from build123d import *

# Parameters (mm, degrees)
CUT_EXTRUDE1_DEPTH = 1.1


with BuildPart() as part:
    # Sketch1 → Revolve1 (revolve)
    with BuildSketch(Plane.XY):
        with BuildLine():
            Line((-2.36, 0), (-2.36, 2))
            Line((-2.36, 2), (-2.11, 2.25))
            Line((-2.11, 2.25), (0, 2.25))
            Line((0, 2.25), (0, 1.35))
            ThreePointArc((0, 1.35), (0.029289322, 1.279289322), (0.1, 1.25))
            Line((0.1, 1.25), (9.7565, 1.25))
            Line((9.7565, 1.25), (10, 1.0065))
            Line((10, 1.0065), (10, 0))
            Line((10, 0), (-2.36, 0))
        make_face()
    revolve(axis=Axis((10, 0, 0), (-1, 0, 0)))

    # Sketch2 → Cut-Extrude1 (cut)
    with BuildSketch(Plane(origin=(-2.36, 0, 0), x_dir=(0, 0, -1), z_dir=(1, 0, 0))):
        Polygon((-1, 0.577350269), (-1, -0.577350269), (0, -1.154700538), (1, -0.577350269), (1, 0.577350269), (0, 1.154700538), align=None)
    extrude(amount=CUT_EXTRUDE1_DEPTH, mode=Mode.SUBTRACT)

    # Sketch3 → Cut-Revolve1 (revolve, cut)
    with BuildSketch(Plane.XY):
        Polygon((-1.26, 0), (-1.26, 1), (-0.682649731, 0), align=None)
    revolve(axis=Axis((-0.682649731, 0, 0), (-1, 0, 0)), mode=Mode.SUBTRACT)


solid = part.part
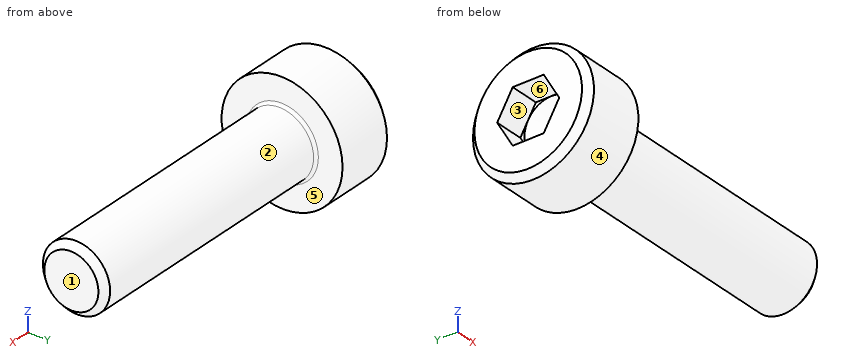
Could you check a few things on this model? Use its own coordinates, in mm. Face numbers are marked on the shaded views. A direction names the side the tool comes from. Round coordinates to 2 decimals unless told otherwise and drop trailing zeros. Write each loop counter-clockwise with the first axis right and the second up, starting at its lowest first coordinate (ties: lowest second). Pieces come first, ordered by that corner, then holes. Notation, with made-up numbers: (69.25, -28) -> (114.25, -28) arc R16 ccw to (114.25, -9) -> close; hole circle Ø7 at (31, 46.5). An arc over 180 degrees is marked (long way). Use a Markdown table: item, result.
1. Please list where these lines run through material, in increasing order: probe 1 along X at (y, z) = (0.8, 1.4); probe 2 along Z at (x, y) = (3.25, 0); probe 3 along Y at (x, z) = (-1.5, 0.15) (3 decimals).
Answer key:
| item | result |
|---|---|
| probe 1 | x = -2.36 to 0 |
| probe 2 | z = -1.25 to 1.25 |
| probe 3 | y = -2.245 to -1.068, 1.068 to 2.245 |
2. If we section it at A-A (x = 1): List the corners of the cut face in (y, z) for me.
Answer key:
| item | result |
|---|---|
| outline | circle Ø2.5 at (0, 0) |
3. Which directions (+Z, -Z, +X, -X, +Y, -Y) give clear straight access to the entire face, cutting with the end or side of a thin tool? Please do the marked faces 4, 5 and 6.
Answer key:
| item | result |
|---|---|
| face 4 | +X, -X |
| face 5 | +X |
| face 6 | -X |
4. We'd pull the mould along Z, two halves only. Please class the marked faces 1, 2 and 3: +Z half, -Z half, draft (parallel to the pull), parting line (faces both ways), or undercut.
Answer key:
| item | result |
|---|---|
| face 1 | draft |
| face 2 | parting line |
| face 3 | undercut |
5. For pin 1 Ø1.5 at (x, y) = (1.5, -1.5) entering from -Z; pin 2 Ø2 at (x, y) = (4.5, -1) entering from -Z, each with a flat end and sliding along its axis, tell me the tip position at first contact or that it passes through.
Answer key:
| item | result |
|---|---|
| pin 1 | stops at z = -1 |
| pin 2 | stops at z = -1.25 |
